For this review, take the finished solid that the model builds, in its own axes (mm). A direction names the side the tool comes from. Coordinates: 2 decimals unless noted, no trailing zeros. Loops run counter-clockwise (first coordinate to the right, second up) from the corner with the lowest first, then second, coordinate; pieces in that order, holes last. Notation, with made-up numbers: M 31,-11.5 L 89,-11.5 A23 ccw 89,0.5 Z; hole C -26.75,52 d4. An arc over 180 degrees is marked long. Answer as a JSON object with one key per item and string values. Group by question number.
Item 1: Mouldability with a two-part tool opening along Z and no side actions: class faces 1 (the face through (45, 2, -1)), 2 (the face through (-36.99, 0.07, -32.15)), 3 (the face through (0, 0, 45)) as +Z half, -Z half, draft (parallel to the pull), parting line (faces both ways), or undercut.
Item 2: Insertion check: pin 1 (3 mm diameter, centred on y = 0, z = -40, fed in from -X); pin 2 (3 mm diameter, centred on x = -23.5, y = 3, fed in from +Z). Each pin has a flat end and moves straight along its axis. Give the tip position at first contact, or say it passes through.
Item 3: Tool access review of faces 4 (the face through (36.57, -0.07, 38.35)), 5 (the face through (0, 0, -35)), 6 (the face through (38, 0, -46)), 7 (the face through (-42, 0, 60)), 8 (the face through (-40, 0.1, 57.2)): name each direction out of +Z, -Z, +X, -X, +Y, -Y from which nothing blocks a thin tool from reaching the whole face with its end or side.
Item 4: Wall thickness on L1, parallel to Z at x = -6, y = 3.5; L2, parallel to Y at x = -37.75, z = 40; L3, parallel to X at y = -1.25, z = 52.5: over which ranges is each line inside the solid? List them lowest first. Write a range as from..to.
Item 5: Add section A-A (x = -20). State the section outline as (y, z) points, then the cut area to 3 significant figures.
Item 6: Add section D-D (x = 19.5). State the section outline as (y, z) points.
Item 7: Add section B-B (z = 31). State the section outline as (x, y) points, then the cut area to 3 significant figures.
Item 8: Add section C-C (z = -26.5). State the section outline as (x, y) points.
from build123d import *

# Parameters (mm, degrees)
EXTRUDE_1_DEPTH             = 5
SKETCH_2_R                  = 2.05
CUT_EXTRUDE_1_DEPTH         = 109.282039139
HOLE_WIZARD_M4_2_AT_2_COUNT = 2
HOLE_WIZARD_M4_2_AT_2_PITCH = 40
HOLE_WIZARD_M4_2_AT_3_COUNT = 2
HOLE_WIZARD_M4_2_AT_3_PITCH = 40
FILLET_1_R                  = 5
HOLE_WIZARD_M5_1_D          = 4.2


with BuildPart() as part:
    # 草图1 → 凸台-拉伸1 (new, symmetric)
    with BuildSketch(Plane(origin=(0, 0, 0), x_dir=(1, 0, 0), z_dir=(0, 1, 0))):
        Polygon((-45, 60), (-40, 60), (-40, 45), (40, 45), (40, 60), (45, 60), (45, -60), (40, -60), (40, -45), (-40, -45), (-40, -60), (-45, -60), align=None)
        with BuildLine():
            Line((-30, 5), (30, 5))
            ThreePointArc((30, 5), (37.071067812, 7.928932188), (40, 15))
            Line((40, 15), (40, 25))
            ThreePointArc((40, 25), (37.071067812, 32.071067812), (30, 35))
            Line((30, 35), (-30, 35))
            ThreePointArc((-30, 35), (-37.071067812, 32.071067812), (-40, 25))
            Line((-40, 25), (-40, 15))
            ThreePointArc((-40, 15), (-37.071067812, 7.928932188), (-30, 5))
        make_face(mode=Mode.SUBTRACT)
        with BuildLine():
            Line((30, -5), (-30, -5))
            ThreePointArc((-30, -5), (-37.071067812, -7.928932188), (-40, -15))
            Line((-40, -15), (-40, -25))
            ThreePointArc((-40, -25), (-37.071067812, -32.071067812), (-30, -35))
            Line((-30, -35), (30, -35))
            ThreePointArc((30, -35), (37.071067812, -32.071067812), (40, -25))
            Line((40, -25), (40, -15))
            ThreePointArc((40, -15), (37.071067812, -7.928932188), (30, -5))
        make_face(mode=Mode.SUBTRACT)
    extrude(amount=EXTRUDE_1_DEPTH, both=True)

    # 草图2 → 切除-拉伸1 (cut, through all)
    with BuildSketch(Plane.ZY.offset(45)):
        with Locations((-55, 0)):
            Circle(SKETCH_2_R)
        with Locations((55, 0)):
            Circle(SKETCH_2_R)
        with Locations((-20, 0)):
            Circle(SKETCH_2_R)
        with Locations((20, 0)):
            Circle(SKETCH_2_R)
    extrude(amount=-CUT_EXTRUDE_1_DEPTH, mode=Mode.SUBTRACT)

    # 草图6 → M4 螺纹孔2 (revolve, cut)
    with BuildSketch(Plane(origin=(-45, 0, 0), x_dir=(0, 0, 1), z_dir=(0, 1, 0))):
        Polygon((0, 0), (0, 18.091420021), (1.65, 17.1), (1.65, 0), align=None)
    hole_wizard_m4_2 = revolve(axis=Axis((-51.35, 0, 0), (1, 0, 0)), mode=Mode.SUBTRACT)

    # M4 螺纹孔2 at 2: M4 螺纹孔2 ×2
    with Locations(*[(0, 0, -i * HOLE_WIZARD_M4_2_AT_2_PITCH) for i in range(1, HOLE_WIZARD_M4_2_AT_2_COUNT)]):
        add(hole_wizard_m4_2, mode=Mode.SUBTRACT)

    # M4 螺纹孔2 at 3: M4 螺纹孔2 ×2
    with Locations(*[(0, 0, i * HOLE_WIZARD_M4_2_AT_3_PITCH) for i in range(1, HOLE_WIZARD_M4_2_AT_3_COUNT)]):
        add(hole_wizard_m4_2, mode=Mode.SUBTRACT)

    # 镜向1: M4 螺纹孔2 across plane
    add(hole_wizard_m4_2.mirror(Plane(origin=(0, 0, 0), x_dir=(0, 0, 1), z_dir=(1, 0, 0))), mode=Mode.SUBTRACT)

    # 镜向1 copy 1 sketch → 镜向1 copy 1 (revolve, cut)
    with BuildSketch(Plane(origin=(45, 0, -40), x_dir=(0, 0, 1), z_dir=(0, 1, 0))):
        Polygon((0, 0), (0, -18.091420021), (1.65, -17.1), (1.65, 0), align=None)
    revolve(axis=Axis((51.35, 0, -40), (1, 0, 0)), mode=Mode.SUBTRACT)

    # 镜向1 copy 2 sketch → 镜向1 copy 2 (revolve, cut)
    with BuildSketch(Plane(origin=(45, 0, 40), x_dir=(0, 0, 1), z_dir=(0, 1, 0))):
        Polygon((0, 0), (0, -18.091420021), (1.65, -17.1), (1.65, 0), align=None)
    revolve(axis=Axis((51.35, 0, 40), (1, 0, 0)), mode=Mode.SUBTRACT)

    # 圆角1
    fillet_1_edges = [part.edges().sort_by_distance(p)[0] for p in [
        (-40, 0, -45),
        (40, 0, -45),
        (40, 0, 45),
        (-40, 0, 45),
    ]]
    fillet(fillet_1_edges, radius=FILLET_1_R)

    # M5 螺纹孔1 (through all)
    with Locations(Plane(origin=(0, 5, 0), x_dir=(1, 0, 0), z_dir=(0, 1, 0))):
        with Locations((20, 40), (20, 0), (20, -40), (-20, -40), (-20, 0), (-20, 40)):
            Hole(HOLE_WIZARD_M5_1_D / 2)


solid = part.part
From the geometry:
{
 "1": {"face 1": "draft", "face 2": "undercut", "face 3": "+Z half"},
 "2": {"pin 1": "stops at x = -27.81", "pin 2": "stops at z = 45"},
 "3": {"face 4": "+X", "face 5": "+Y, -Y", "face 6": "-Z, +Y, -Y", "face 7": "+Z, +X, -X, +Y, -Y", "face 8": "+Z, +Y, -Y"},
 "4": {"L1": "z = -45..-35, -5..5, 35..45", "L2": "y = -5..-1.65, 1.65..5", "L3": "x = -45..-40, 40..45"},
 "5": {"outline": "M -5,-45 L 5,-45 L 5,-42.1 L -5,-42.1 Z; M -5,-37.9 L 5,-37.9 L 5,-35 L -5,-35 Z; M -5,-5 L 5,-5 L 5,-2.1 L -5,-2.1 Z; M -5,2.1 L 5,2.1 L 5,5 L -5,5 Z; M -5,35 L 5,35 L 5,37.9 L -5,37.9 Z; M -5,42.1 L 5,42.1 L 5,45 L -5,45 Z", "area": "174 mm²"},
 "6": {"outline": "M -5,-45 L 5,-45 L 5,-42.04 L -5,-42.04 Z; M -5,-37.96 L 5,-37.96 L 5,-35 L -5,-35 Z; M -5,-5 L 5,-5 L 5,-2.04 L -5,-2.04 Z; M -5,2.04 L 5,2.04 L 5,5 L -5,5 Z; M -5,35 L 5,35 L 5,37.96 L -5,37.96 Z; M -5,42.04 L 5,42.04 L 5,45 L -5,45 Z"},
 "7": {"outline": "M -45,-5 L -38,-5 L -38,5 L -45,5 Z; M 38,-5 L 45,-5 L 45,5 L 38,5 Z", "area": "140 mm²"},
 "8": {"outline": "M -45,-5 L -39.89,-5 L -39.89,5 L -45,5 Z; M 39.89,-5 L 45,-5 L 45,5 L 39.89,5 Z"}
}
